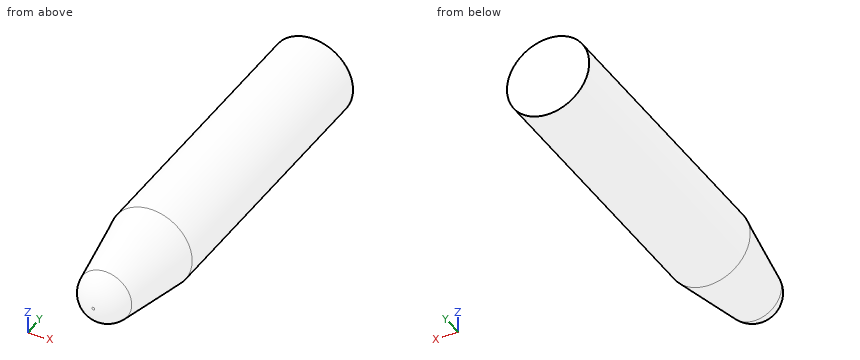
```python
from build123d import *

# Parameters (mm, degrees)
F0_R     = 2.25
F1_DEPTH = 21.5
F2_SIZE2 = 1
F2_SIZE  = 5.6712818196
F3_R     = 1.4


with BuildPart() as f1:
    # F0 (on Front) → F1 (new body)
    with BuildSketch(Plane.XZ):
        Circle(F0_R)
    extrude(amount=F1_DEPTH)

    # F2
    f2_edges = [f1.edges().sort_by_distance(p)[0] for p in [
        (-2.25, -21.5, 0),
    ]]
    f2_side = f1.faces().sort_by_distance((-2.25, -10.75, 0))[0]
    chamfer(f2_edges, length=F2_SIZE, length2=F2_SIZE2, reference=f2_side)

    # F3
    f3_edges = [f1.edges().sort_by_distance(p)[0] for p in [
        (-1.25, -21.5, 0),
    ]]
    fillet(f3_edges, radius=F3_R)


solid = f1.part
```
Here's how the part is built. I have some questions about the finished solid (model axes, mm). Coordinates: 2 decimals unless noted, no trailing zeros. Write each loop counter-clockwise with the first axis right and the second up, starting at its lowest first coordinate (ties: lowest second). Pieces come first, ordered by that corner, then holes. Notation, with made-up numbers: (2.5, 52) -> (39.5, 52) arc R25 cw to (39.5, 80) -> close; hole circle Ø2 at (86.5, -34). An arc over 180 degrees is marked (long way). Use a Markdown table: item, result. Add a question column.
(1) Please list where these lines run through material, in increasing order: line 1 (Z direction, x = 1, y = -9.25); line 2 (Z direction, x = 1.55, y = -5.5); line 3 (X direction, y = -1.5, z = 1.45).
(2) I'm going to push a flat-ended pin straight in: P1, Ø1, axis at y = -13.5, z = 1, coming from the -X side. Where does the tip first touch, or does it pass through?
(3) If we section it at A-A, the plane y = -10: Write out the boundary of the cut face in (x, z), and give its area (3 significant figures).
Outcome:
| question | item | result |
|---|---|---|
| 1 | line 1 | z = -2.02 to 2.02 |
| 1 | line 2 | z = -1.63 to 1.63 |
| 1 | line 3 | x = -1.72 to 1.72 |
| 2 | P1 | stops at x = -2.19 |
| 3 | outline | circle Ø4.5 at (0, 0) |
| 3 | area | 15.9 mm^2 |
